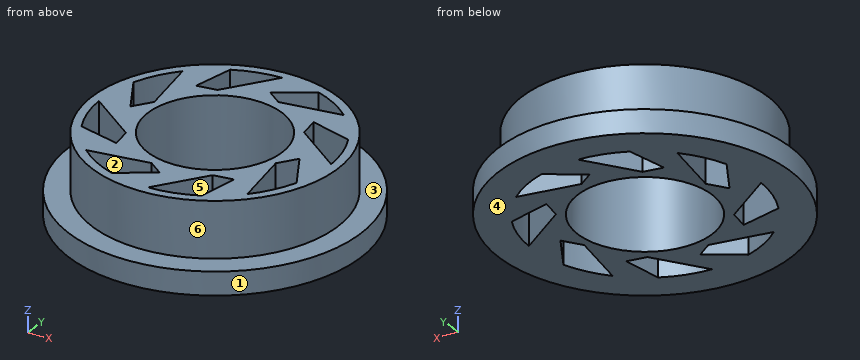
from build123d import *

# Parameters (mm, degrees)
F0_R     = 26.5
F0_R_2   = 14.5
F1_DEPTH = 17
F0_R_3   = 31.5
F2_DEPTH = 5
F3_DEPTH = 17


with BuildPart() as f1:
    # F0 (on Top) → F1 (new body)
    with BuildSketch(Plane.XY):
        Circle(F0_R)
        with BuildLine():
            Line((-3.216465, -16.254543), (0, -18.5))
            Line((0, -18.5), (-7.269078, -23.451694))
            ThreePointArc((-7.269078, -23.451694), (-11.892593, -21.479937), (-16.01768, -18.607939))
            Line((-16.01768, -18.607939), (-3.216465, -16.254543))
        make_face(mode=Mode.SUBTRACT)
        with BuildLine():
            Line((-13.598169, -9.006938), (-12.86031, -13.298963))
            Line((-12.86031, -13.298963), (-21.752187, -11.387001))
            ThreePointArc((-21.752187, -11.387001), (-23.666893, -6.534493), (-24.513214, -1.387001))
            Line((-24.513214, -1.387001), (-13.598169, -9.006938))
        make_face(mode=Mode.SUBTRACT)
        with BuildLine():
            Line((8.679206, -14.067624), (12.86031, -13.298963))
            Line((12.86031, -13.298963), (11.387001, -21.752187))
            ThreePointArc((11.387001, -21.752187), (6.534493, -23.666893), (1.387001, -24.513214))
            Line((1.387001, -24.513214), (8.679206, -14.067624))
        make_face(mode=Mode.SUBTRACT)
        with BuildLine():
            Line((15.809209, -3.854376), (18.5, 0))
            Line((18.5, 0), (23.172504, -8.115203))
            ThreePointArc((23.172504, -8.115203), (21.034287, -12.664131), (18.014507, -16.682295))
            Line((18.014507, -16.682295), (15.809209, -3.854376))
        make_face(mode=Mode.SUBTRACT)
        with BuildLine():
            Line((-15.809209, 3.854376), (-18.5, 0))
            Line((-18.5, 0), (-23.172504, 8.115203))
            ThreePointArc((-23.172504, 8.115203), (-21.034287, 12.664131), (-18.014507, 16.682295))
            Line((-18.014507, 16.682295), (-15.809209, 3.854376))
        make_face(mode=Mode.SUBTRACT)
        with BuildLine():
            Line((-8.679206, 14.067624), (-12.86031, 13.298963))
            Line((-12.86031, 13.298963), (-11.04677, 21.926931))
            ThreePointArc((-11.04677, 21.926931), (-6.349952, 23.717073), (-1.387001, 24.513214))
            Line((-1.387001, 24.513214), (-8.679206, 14.067624))
        make_face(mode=Mode.SUBTRACT)
        Circle(F0_R_2, mode=Mode.SUBTRACT)
        with BuildLine():
            Line((13.598169, 9.006938), (12.86031, 13.298963))
            Line((12.86031, 13.298963), (21.926931, 11.04677))
            ThreePointArc((21.926931, 11.04677), (23.717073, 6.349952), (24.513214, 1.387001))
            Line((24.513214, 1.387001), (13.598169, 9.006938))
        make_face(mode=Mode.SUBTRACT)
        with BuildLine():
            Line((3.216465, 16.254543), (0, 18.5))
            Line((0, 18.5), (7.269078, 23.451694))
            ThreePointArc((7.269078, 23.451694), (11.892593, 21.479937), (16.01768, 18.607939))
            Line((16.01768, 18.607939), (3.216465, 16.254543))
        make_face(mode=Mode.SUBTRACT)
    extrude(amount=F1_DEPTH)

    # F0 (on Top) → F2 (join)
    with BuildSketch(Plane.XY):
        Circle(F0_R_3)
        Circle(F0_R, mode=Mode.SUBTRACT)
    extrude(amount=F2_DEPTH)

    # F0 (on Top) → F3 (cut)
    with BuildSketch(Plane.XY):
        with BuildLine():
            Line((23.172504, -8.115203), (18.5, 0))
            Line((18.5, 0), (15.809209, -3.854376))
            Line((15.809209, -3.854376), (18.014507, -16.682295))
            ThreePointArc((18.014507, -16.682295), (21.034287, -12.664131), (23.172504, -8.115203))
        make_face()
        with BuildLine():
            Line((11.387001, -21.752187), (12.86031, -13.298963))
            Line((12.86031, -13.298963), (8.679206, -14.067624))
            Line((8.679206, -14.067624), (1.387001, -24.513214))
            ThreePointArc((1.387001, -24.513214), (6.534493, -23.666893), (11.387001, -21.752187))
        make_face()
        with BuildLine():
            Line((-7.269078, -23.451694), (0, -18.5))
            Line((0, -18.5), (-3.216465, -16.254543))
            Line((-3.216465, -16.254543), (-16.01768, -18.607939))
            ThreePointArc((-16.01768, -18.607939), (-11.892593, -21.479937), (-7.269078, -23.451694))
        make_face()
        with BuildLine():
            Line((-21.752187, -11.387001), (-12.86031, -13.298963))
            Line((-12.86031, -13.298963), (-13.598169, -9.006938))
            Line((-13.598169, -9.006938), (-24.513214, -1.387001))
            ThreePointArc((-24.513214, -1.387001), (-23.666893, -6.534493), (-21.752187, -11.387001))
        make_face()
        with BuildLine():
            Line((-23.172504, 8.115203), (-18.5, 0))
            Line((-18.5, 0), (-15.809209, 3.854376))
            Line((-15.809209, 3.854376), (-18.014507, 16.682295))
            ThreePointArc((-18.014507, 16.682295), (-21.034287, 12.664131), (-23.172504, 8.115203))
        make_face()
        with BuildLine():
            Line((-11.04677, 21.926931), (-12.86031, 13.298963))
            Line((-12.86031, 13.298963), (-8.679206, 14.067624))
            Line((-8.679206, 14.067624), (-1.387001, 24.513214))
            ThreePointArc((-1.387001, 24.513214), (-6.349952, 23.717073), (-11.04677, 21.926931))
        make_face()
        with BuildLine():
            Line((7.269078, 23.451694), (0, 18.5))
            Line((0, 18.5), (3.216465, 16.254543))
            Line((3.216465, 16.254543), (16.01768, 18.607939))
            ThreePointArc((16.01768, 18.607939), (11.892593, 21.479937), (7.269078, 23.451694))
        make_face()
        with BuildLine():
            Line((21.926931, 11.04677), (12.86031, 13.298963))
            Line((12.86031, 13.298963), (13.598169, 9.006938))
            Line((13.598169, 9.006938), (24.513214, 1.387001))
            ThreePointArc((24.513214, 1.387001), (23.717073, 6.349952), (21.926931, 11.04677))
        make_face()
    extrude(amount=F3_DEPTH, mode=Mode.SUBTRACT)


solid = f1.part
Source: CAD feature listing. Evaluate the final solid. Frame: model axes, mm. Face numbers are marked on the shaded views. A direction names the side the tool comes from. Coordinates: 2 decimals unless noted, no trailing zeros. Order: outer loops, then holes, each group sorted by start corner. A loop starts at its lowest first (then second) coordinate and runs counter-clockwise, first axis right, second up.
Item 1: Cut plane A-A (y = 21). Return loops of the section in (x, z).
Output values:
outline: (-23.48, 0) - (-11.24, 0) - (-11.24, 17) - (-16.16, 17) - (-16.16, 5) - (-23.48, 5) - close; (-3.84, 0) - (3.67, 0) - (3.67, 17) - (-3.84, 17) - close; (12.72, 0) - (23.48, 0) - (23.48, 5) - (16.16, 5) - (16.16, 17) - (12.72, 17) - close
Item 2: Set-up query: the marked faces 4, 5 and 6. Return all of +Z, -Z, +X, -X, +Y, -Y with unobstructed straight access to the full face (end or side cutting, diameter ignored); none if empty.
Output values:
face 4: -Z, +X, -X, +Y, -Y
face 5: +Z, -Z
face 6: +Z
Item 3: Material intervals for line 1 (Y direction, x = -9.5, z = 14); line 2 (Y direction, x = 21, z = 10); line 3 (Y direction, x = -9, z = 14), sorted ascending.
Output values:
line 1: y = -24.74 to -22.64, -17.41 to -10.95, 10.95 to 13.92, 22.64 to 24.74
line 2: y = -16.16 to -12.72, -4.34 to 3.84, 11.28 to 16.16
line 3: y = -24.92 to -22.84, -17.32 to -11.37, 11.37 to 14.01, 22.84 to 24.92
Item 4: Cut plane D-D (y = -20.5). Return loops of the section in (x, z), plus the area to 3 significant figures.
Output values:
outline: (-23.92, 0) - (-13.51, 0) - (-13.51, 17) - (-16.79, 17) - (-16.79, 5) - (-23.92, 5) - close; (-2.94, 0) - (4.19, 0) - (4.19, 17) - (-2.94, 17) - close; (11.61, 0) - (23.92, 0) - (23.92, 5) - (16.79, 5) - (16.79, 17) - (11.61, 17) - close
area: 336 mm2
Item 5: Pull-direction query (Y, two-part tool) for the marked faces 1, 2 and 3; classes: pulls with the +Y half, pulls with the -Y half, needs draft (parallel to the pull), parting line crosses it, or undercut.
Output values:
face 1: parting line crosses it
face 2: undercut
face 3: needs draft
Item 6: First-contact query: P1, Ø5, axis at y = 16.5, z = 8.5, coming from the +X side; P2, Ø10, axis at y = -12, z = 8, coming from the +X side; P3, Ø1.5, axis at y = 16, z = 5.5, coming from the -X side. Flat tips, straight axial feed; report the tip coordinate or a pass-through.
Output values:
P1: stops at x = 22.5
P2: stops at x = 30.47
P3: stops at x = -27.46
Item 7: Cut plane B-B (x = 5.5). Return loops of the section in (y, z).
Output values:
outline: (-31.02, 0) - (-23.93, 0) - (-23.93, 17) - (-25.92, 17) - (-25.92, 5) - (-31.02, 5) - close; (-18.62, 0) - (-13.42, 0) - (-13.42, 17) - (-18.62, 17) - close; (13.42, 0) - (16.67, 0) - (16.67, 17) - (13.42, 17) - close; (22.25, 0) - (31.02, 0) - (31.02, 5) - (25.92, 5) - (25.92, 17) - (22.25, 17) - close
Item 8: Cut plane C-C (z = 5.75). Count the separate pieces of the cut face and the enclosed holes in it, plus the area to 3 significant figures.
Output values:
separate pieces: 1
enclosed holes: 9
area: 1,040 mm2
